Job drawing, mm, ordinate dimensions from the low corner. One solid piece. A direction names the side the tool comes from. Coordinates: 2 decimals unless noted, no trailing zeros. Write each loop counter-clockwise with the first axis right and the second up, starting at its lowest first coordinate (ties: lowest second). Pieces come first, ordered by that corner, then holes.
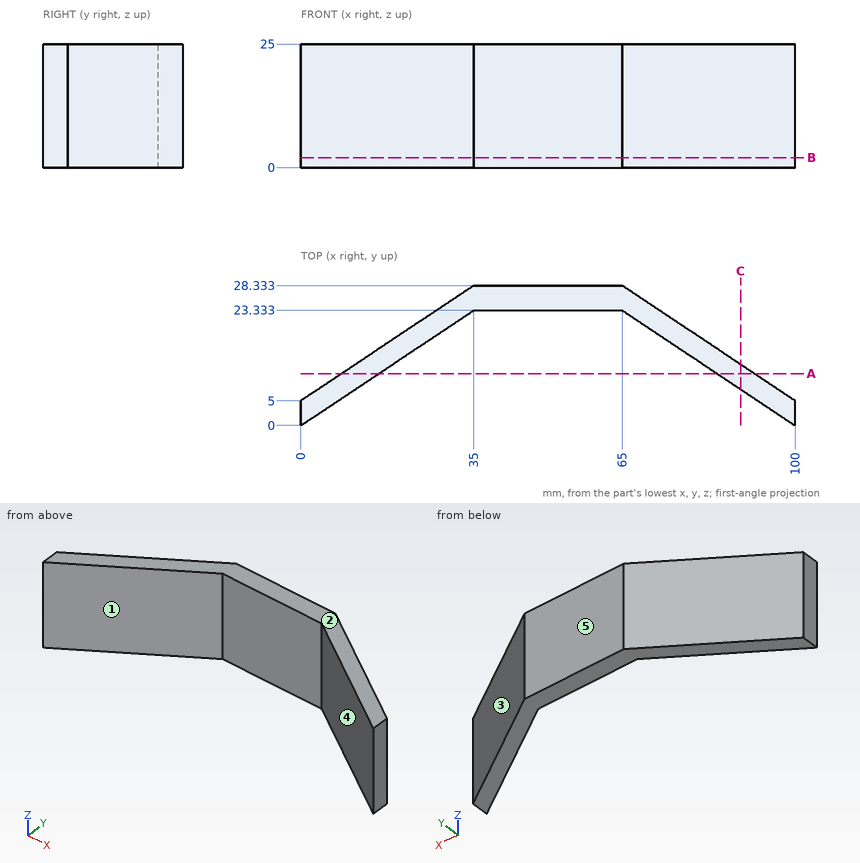
1. Saw through at C-C on x = 89. List the corners of the cut face in (y, z), plus the area to 3 significant figures.
Computed values:
outline: (7.33, 0) - (12.33, 0) - (12.33, 25) - (7.33, 25) - close
area: 125 mm2
2. Probe line 1 along Y through (x, z) = (55, 11.75); line 2 along X through (y, z) = (7.75, 15.25) (1 decimal); line 3 along X through (y, z) = (2, 23). List the from-to ranges inside material, lowest first.
Computed values:
line 1: y = 23.33 to 28.33
line 2: x = 4.1 to 11.6, 88.4 to 95.9
line 3: x = 0 to 3, 97 to 100
3. Flat gauge pins, fed straight in: pin 1 (4 mm diameter, centred on y = 17.5, z = 6.5, fed in from +X); pin 2 (12.5 mm diameter, centred on x = 43, z = 14, fed in from -Y); pin 3 (8 mm diameter, centred on y = 23.5, z = 15.5, fed in from -X). Where does each tip first touch, or does it go through?
Computed values:
pin 1: stops at x = 84.25
pin 2: stops at y = 23.33
pin 3: stops at x = 21.75
4. 3-axis set-ups, long thin cutter, end or side, ignore diameter. For the marked faces 4 and 5: which of +Z, -Z, +X, -X, +Y, -Y reach the whole face in a straight line?
Computed values:
face 4: +Z, -Z, -Y
face 5: +Z, -Z, +X, -X, +Y
5. Saw through at A-A on y = 10.5. List the corners of the cut face in (x, z), plus the area to 3 significant figures.
Computed values:
outline: (8.25, 0) - (15.75, 0) - (15.75, 25) - (8.25, 25) - close; (84.25, 0) - (91.75, 0) - (91.75, 25) - (84.25, 25) - close
area: 375 mm2
6. Mould opens along X. For the marked faces 1, 2 and 3 say: +X half, -X half, draft (parallel to the pull), parting line (faces both ways), or undercut.
Computed values:
face 1: undercut
face 2: draft
face 3: +X half
7. Saw through at B-B on z = 2. List the corners of the cut face in (x, y), plus the area to 3 significant figures.
Computed values:
outline: (0, 0) - (35, 23.33) - (65, 23.33) - (100, 0) - (100, 5) - (65, 28.33) - (35, 28.33) - (0, 5) - close
area: 500 mm2
